Verification items for the finished model (mm, model axes). A direction names the side the tool comes from. Round coordinates to 2 decimals unless told otherwise and drop trailing zeros. Write each loop counter-clockwise with the first axis right and the second up, starting at its lowest first coordinate (ties: lowest second). Pieces come first, ordered by that corner, then holes. Notation, with made-up numbers: M -13,29 L 2,29 A14 cw 2,54 Z; hole C 61.5,-15 d11. An arc over 180 degrees is marked long. Use a Markdown table: item, result. Add a question column.
Autodesk Inventor part; units mm, degrees
ref_plane "Arbeitsebene2" through (2.5, 0, 3.75) normal (1, 0, 0) x (0, 1, 0)
ref_plane "XZ Plane" through (0, 0, 0) normal (0, 1, 0) x (-1, 0, 0)
ref_plane "XY Plane" through (0, 0, 0) normal (0, 0, 1) x (1, 0, 0)
sketch "Skizze1" plane through (0, 0, 0) normal (0, 1, 0) x (-1, 0, 0)
  line L0 (0, 0) -> (0, 9)
  line L1 (0, 0) -> (2.9, 0)
  line L2 (2.9, 0) -> (2.9, 1)
  line L3 (2.9, 1) -> (2.5, 1)
  line L4 (2.5, 1) -> (2.5, 6.5)
  arc A0 (2.5, 6.5) -> (0, 9) centre (0, 6.5) ccw
  dimension "d0" = 5.8
  dimension "d2" = 5
  dimension "d3" = 9
  dimension "d4" = 1
revolve "Umdrehung1" add sketch "Skizze1" angle 360 about axis through (0, 0, 0) along (0, 0, 1)
ref_plane "Arbeitsebene2" through (2.5, 0, 3.75) normal (1, 0, 0) x (0, 1, 0)
sketch "Skizze2" plane through (2.5, 0, 3.75) normal (1, 0, 0) x (0, 1, 0)
  line L0 (-2.9, -3.75) -> (2.9, -3.75)
  line L1 (-2.9, -2.75) -> (2.9, -2.75)
  line L2 (-2.9, -2.75) -> (2.9, -2.75)
  line L3 (2.9, -2.75) -> (2.9, -3.75)
  line L4 (2.9, -3.75) -> (-2.9, -3.75)
  line L5 (-2.9, -3.75) -> (-2.9, -2.75)
  point P0 (0, -3.75)
extrude "Extrusion1" cut sketch "Skizze2" along normal blind 1
sketch "Skizze3" plane through (0, 0, 0) normal (0, 0, -1) x (-1, 0, 0)
  line L0 (-1.5, 0.225) -> (-1, 0.225)
  line L1 (-1, 0.225) -> (-1, -0.225)
  line L2 (-1, -0.225) -> (-1.5, -0.225)
  line L3 (-1.5, -0.225) -> (-1.5, 0.225)
  line L4 (1, 0.225) -> (1.5, 0.225)
  line L5 (1.5, 0.225) -> (1.5, -0.225)
  line L6 (1.5, -0.225) -> (1, -0.225)
  line L7 (1, -0.225) -> (1, 0.225)
  line L8 (0, -4.06) -> (0, 4.06)
  line L9 (-3.58, 0) -> (3.98, 0)
  point P0 (0, 0)
  dimension "d8" = 0.5
  dimension "d10" = 0.45
  dimension "d11" = 3
extrude "Extrusion2" add sketch "Skizze3" along normal blind 5
sketch "Skizze4" plane through (1, -0.225, 0) normal (0, -1, 0) x (1, 0, 0)
  line L0 (1.4937, -1) -> (-4.2917, -1)
  line L1 (-3.9, 0) -> (1.5, 0)
  point P0 (-1, 0)
  dimension "d14" = 1
bend part "Biegungsteil1" radius 1.4324 angle 40 line through (2.4937, -0.225, -1) along (-1, 0, 0) centre toward (0, -1, 0) moving side (0, 0, -1) both sides no
properties part number "LED 5mm" material "PC/ABS-Kunststoff"
1. Cross-section at C-C on y = -1.6. Enter the section's corners in (x, z).
2. Cross-section at A-A on z = -0.25. Enter the section's corners in (x, y) (3 decimals).
3. Release check for a two-part mould opening along Z. For faces 1 (the flat face through (1.25, -1.51, -3.05)), 2 (the flat face through (-1.5, -0.7, -2.4)), 3 (the flat face through (-1.246, -1.166, -3.343)) record: +Z half, -Z half, draft (parallel to the pull), parting line (faces both ways), or undercut.
4. Cross-section at B-B on x = 0. Enter the section's corners in (y, z), plus the area to 3 significant figures.
5. Scan lines: line 1 along Y through (x, z) = (-0.1, 6.25); line 2 along Z through (x, y) = (2.1, -1.85); line 3 along Z through (x, y) = (-1.35, -1). Record each from-to range of solid material in increasing order. Write a range as from..to.
6. Cross-section at D-D on y = 2.15. Enter the section's corners in (x, z).
7. Access from +Z, -Z, +X, -X, +Y, -Y to the whole of each face (thin tool, end or side, straight path). Record for faces 4 (the flat face through (1.5, -0.8, -2.6)), 5 (the flat face through (1, -0.7, -2.4)), 6 (the cylindrical face through (0.54, 2.44, 3.79)), 7 (the flat face through (-1.25, -1.51, -3.05)).
8. Depth check by flat-ended pin: pin 1 Ø2 at (y, z) = (-1, -3.5) entering from +X; pin 2 Ø2 at (y, z) = (-1.5, -2) entering from -X; pin 3 Ø2 at (y, z) = (-2, 2.5) entering from +X. Enter the tip coordinate at first touch or a pass-through.
Answer:
| question | item | result |
|---|---|---|
| 1 | outline | M -2.42,0 L 2.42,0 L 2.42,1 L 1.92,1 L 1.92,6.5 A1.92 ccw -1.92,6.5 L -1.92,1 L -2.42,1 Z; M -1.5,-3.86 L -1,-3.86 L -1,-3.16 L -1.5,-3.16 Z; M 1,-3.86 L 1.5,-3.86 L 1.5,-3.16 L 1,-3.16 Z |
| 2 | outline | M -1.5,-0.225 L -1,-0.225 L -1,0.225 L -1.5,0.225 Z; M 1,-0.225 L 1.5,-0.225 L 1.5,0.225 L 1,0.225 Z |
| 3 | face 1 | undercut |
| 3 | face 2 | draft |
| 3 | face 3 | -Z half |
| 4 | outline | M -2.9,0 L 2.9,0 L 2.9,1 L 2.5,1 L 2.5,6.5 A2.5 ccw -2.5,6.5 L -2.5,1 L -2.9,1 Z |
| 4 | area | 43.1 mm^2 |
| 5 | line 1 | y = -2.5..2.5 |
| 5 | line 2 | z = 0..1 |
| 5 | line 3 | z = -3.15..-2.44, 0..8.35 |
| 6 | outline | M -1.95,0 L 1.95,0 L 1.95,1 L 1.28,1 L 1.28,6.5 A1.28 ccw -1.28,6.5 L -1.28,1 L -1.95,1 Z |
| 7 | face 4 | -Z, +X, +Y, -Y |
| 7 | face 5 | -Z, +Y, -Y |
| 7 | face 6 | +Z |
| 7 | face 7 | +X, -X, -Y |
| 8 | pin 1 | stops at x = 1.5 |
| 8 | pin 2 | stops at x = -1.5 |
| 8 | pin 3 | stops at x = 2.29 |
